Design review of the part built by this model. Coordinates are the model's own, in mm. Give positions to 0.01 mm unless a question says otherwise; leave off trailing zeros. Loops run counter-clockwise (first coordinate to the right, second up) from the corner with the lowest first, then second, coordinate; pieces in that order, holes last. Notation, with made-up numbers: (31.5, -39.5) - (58.5, -39.5) arc R19 ccw to (58.5, -26.5) - close; hole circle Ø9 at (81.25, 57.5). An arc over 180 degrees is marked (long way). One line per item, written item: value. Start each with the question number.
```python
from build123d import *
from build123d.topology import SkipClean

# Parameters (mm, degrees)
SKETCH3_R           = 88.9
BOSS_EXTRUDE1_DEPTH = 457.2
BOSS_EXTRUDE1_DRAFT = -4
FILLET1_R           = 50.8


with BuildPart() as part:
    # Sketch3 → Boss-Extrude1 (with draft: the straight prism first)
    with BuildSketch(Plane.XY):
        Circle(SKETCH3_R)
    extrude(amount=-BOSS_EXTRUDE1_DEPTH)
    # Boss-Extrude1: the draft: its side faces are tilted about the plane it starts from
    boss_extrude1_sides = [part.faces().sort_by_distance(p)[0] for p in [
        (-88.9, 0, -228.6),
    ]]
    draft(boss_extrude1_sides, Plane.XY, BOSS_EXTRUDE1_DRAFT)

    # Sketch6 → Revolve1 (revolve)
    with SkipClean():  # the faces are left unmerged after this step: merging them gives an invalid solid
        with BuildSketch(Plane(origin=(0, 0, 0), x_dir=(0, 0, -1), z_dir=(1, 0, 0))):
            with BuildLine():
                Line((457.2, -56.929461579), (457.2, 56.929461579))
                ThreePointArc((457.2, 56.929461579), (514.129461579, 0), (457.2, -56.929461579))
            make_face()
        revolve(axis=Axis((0, -56.929461579, -457.2), (0, 1, 0)))

    # Fillet1
    fillet1_edges = [part.edges().sort_by_distance(p)[0] for p in [
        (-88.9, 0, 0),
    ]]
    fillet(fillet1_edges, radius=FILLET1_R)


solid = part.part
```
(1) To check wall thickness, follow L1, parallel to X at y = -43.5, z = -53.5; L2, parallel to X at y = -40.5, z = -333; L3, parallel to Y at x = -38, z = -135.5. State the ranges of each line that lie inside material, in increasing order. Write a range as from..to.
(2) Take a section at B-B on z = -310. State the section outline as (x, y) points.
(3) Take a section at A-A on z = -72.5. State the section outline as (x, y) points, and give its area (3 significant figures).
(4) For pin 1 Ø6 at (x, y) = (45, -11) entering from +Z; pin 2 Ø8 at (x, z) = (54, -86.5) entering from +Y; pin 3 Ø1.5 at (x, z) = (-28.5, -177.5) entering from +Y, all flat-tipped, find the tip position at first contact; note any pin that passes through.
Here are the results:
1. L1: -73.2..73.2
1. L2: -51.62..51.62
1. L3: -69.74..69.74
2. outline: circle Ø134.45 at (0, 0)
3. outline: circle Ø167.66 at (0, 0)
3. area: 22,100 mm²
4. pin 1: z = -0.79
4. pin 2: y = 66.08
4. pin 3: y = 71.28
